```python
from build123d import *

# Parameters (mm, degrees)
F0_R     = 160
F0_R_2   = 140
F1_DEPTH = 50
F0_R_3   = 65
F0_R_4   = 50
F0_R_5   = 30
F0_R_6   = 20
F0_R_7   = 110
F0_R_8   = 90
F3_R     = 160
F4_DEPTH = 25


with BuildPart() as f1:
    # F0 (on Top) → F1 (new body, symmetric)
    with BuildSketch(Plane.XY):
        Circle(F0_R)
        Circle(F0_R_2, mode=Mode.SUBTRACT)
    extrude(amount=F1_DEPTH, both=True)



with BuildPart() as f1b:
    # F0 (on Top) → F1, piece 2 (new body, symmetric)
    with BuildSketch(Plane.XY):
        Circle(F0_R_3)
        Circle(F0_R_4, mode=Mode.SUBTRACT)
    extrude(amount=F1_DEPTH, both=True)


with BuildPart() as f1c:
    # F0 (on Top) → F1, piece 3 (new body, symmetric)
    with BuildSketch(Plane.XY):
        Circle(F0_R_5)
        Circle(F0_R_6, mode=Mode.SUBTRACT)
    extrude(amount=F1_DEPTH, both=True)


with BuildPart() as f1d:
    # F0 (on Top) → F1, piece 4 (new body, symmetric)
    with BuildSketch(Plane.XY):
        Circle(F0_R_7)
        Circle(F0_R_8, mode=Mode.SUBTRACT)
    extrude(amount=F1_DEPTH, both=True)


with BuildPart() as f1_1:
    add(f1.part)

    add(f1b.part)  # F4 merges F1b

    add(f1c.part)  # F4 merges F1c

    add(f1d.part)  # F4 merges F1d
    # F3 (on face) → F4 (join)
    with BuildSketch(Plane(origin=(0, 0, -50), x_dir=(1, 0, 0), z_dir=(0, 0, -1))):
        Circle(F3_R)
    extrude(amount=F4_DEPTH)


solid = f1_1.part
```
Part model, mm, in its own coordinate system. A direction names the side the tool comes from. Give positions to 0.01 mm unless a question says otherwise; leave off trailing zeros. Write each loop counter-clockwise with the first axis right and the second up, starting at its lowest first coordinate (ties: lowest second). Pieces come first, ordered by that corner, then holes. Notation, with made-up numbers: M 21,67 L 27,67 A24 cw 27,91 Z; hole C -5,47.25 d3. An arc over 180 degrees is marked long. Use CSV: the item, a comma, the result in double quotes.
Item 1: Slice it at D-D on y = -95. Write the cut outline in (x, z).
Taken from the geometry:
outline,"M -128.74,-75 L 128.74,-75 L 128.74,50 L 102.83,50 L 102.83,-50 L 55.45,-50 L 55.45,50 L -55.45,50 L -55.45,-50 L -102.83,-50 L -102.83,50 L -128.74,50 Z"
Item 2: Slice it at A-A on z = -15.5. Write the cut outline in (x, y).
Taken from the geometry:
outline,"C 0,0 d320; C 0,0 d220; C 0,0 d130; C 0,0 d60; hole C 0,0 d280; hole C 0,0 d180; hole C 0,0 d100; hole C 0,0 d40"
Item 3: Pin check, flat tips, straight feed: P1, Ø6, axis at y = -116, z = -9.5, coming from the +X side; P2, Ø2, axis at y = 119.5, z = -45.5, coming from the +X side; P3, Ø12, axis at x = 0.5, y = 2, coming from the +Z side. Stop position of each tip, or through.
Taken from the geometry:
P1,"stops at x = 113.27"
P2,"stops at x = 107.51"
P3,"stops at z = -50"
Item 4: Pull direction X, two halves, no side cores. Call faces 1 (the face through (0, 0, -50)), 2 (the face through (-41, -81, 50)): +X half, -X half, draft (parallel to the pull), parting line (faces both ways), or undercut.
Taken from the geometry:
face 1,"undercut"
face 2,"draft"
Item 5: Which spindle directions (+Z, -Z, +X, -X, +Y, -Y) get a long thin tool onto all of the face, cutting with end or side? Do faces 3 (the face through (-84, 72, -50)), 4 (the face through (-2, -2, -75)). Say none if no direction does.
Taken from the geometry:
face 3,"+Z"
face 4,"-Z, +X, -X, +Y, -Y"
Item 6: Drill centre lines: probe 1 along X at (y, z) = (-51, -24.5); probe 2 along Y at (x, z) = (-54, -35); probe 3 along Y at (x, z) = (-76.5, -36.5). Where is each one in solid material? Low to high.
Taken from the geometry:
probe 1,"x = -151.65 to -130.38, -97.46 to -74.16, -40.3 to 40.3, 74.16 to 97.46, 130.38 to 151.65"
probe 2,"y = -150.61 to -129.17, -95.83 to -72, -36.18 to 36.18, 72 to 95.83, 129.17 to 150.61"
probe 3,"y = -140.53 to -117.25, -79.04 to -47.41, 47.41 to 79.04, 117.25 to 140.53"
